Could you check a few things on this model? Use its own coordinates, in mm. Give positions to 0.01 mm unless a question says otherwise; leave off trailing zeros. Write each loop counter-clockwise with the first axis right and the second up, starting at its lowest first coordinate (ties: lowest second). Pieces come first, ordered by that corner, then holes. Notation, with made-up numbers: (-15.75, -15) - (31.25, -15) arc R26 cw to (31.25, 19) - close; hole circle Ø2 at (85, 22). An arc over 180 degrees is marked (long way). Answer in a Markdown table with one row per item.
from build123d import *

# Parameters (mm, degrees)
F0_W     = 175
F0_H     = 40
F1_DEPTH = 15
F3_DEPTH = 50.8
F5_DEPTH = 0.001


# Not quite as in the source:
# - a feature names something its author has since deleted; it is built from what else it names


with BuildPart() as f1:
    # F0 (on Top) → F1 (new body, symmetric)
    with BuildSketch(Plane.XY):
        Rectangle(F0_W, F0_H)
    extrude(amount=F1_DEPTH, both=True)

    # F2 (on face) → F3 (cut)
    with BuildSketch(Plane.XZ.offset(20)):
        with BuildLine():
            ThreePointArc((-87.5, 0), (-83.1066017178, 10.6066017178), (-72.5, 15))
            Line((-72.5, 15), (-87.5, 15))
            Line((-87.5, 15), (-87.5, 0))
        make_face()
        with BuildLine():
            Line((-87.5, -15), (-72.5, -15))
            ThreePointArc((-72.5, -15), (-83.1066017178, -10.6066017178), (-87.5, 0))
            Line((-87.5, 0), (-87.5, -15))
        make_face()
        with BuildLine():
            ThreePointArc((87.5, 0), (83.1066017178, -10.6066017178), (72.5, -15))
            Line((72.5, -15), (87.5, -15))
            Line((87.5, -15), (87.5, 0))
        make_face()
        with BuildLine():
            Line((87.5, 15), (72.5, 15))
            ThreePointArc((72.5, 15), (83.1066017178, 10.6066017178), (87.5, 0))
            Line((87.5, 0), (87.5, 15))
        make_face()
    extrude(amount=-F3_DEPTH, mode=Mode.SUBTRACT)

    # F4 (on face) → F5 (join)
    with BuildSketch(Plane.XZ.offset(20)):
        with BuildLine():
            Line((72, 12.5), (-72, 12.5))
            ThreePointArc((-72, 12.5), (-84.5, 0), (-72, -12.5))
            Line((-72, -12.5), (0, -12.5))
            Line((0, -12.5), (72, -12.5))
            ThreePointArc((72, -12.5), (84.5, 0), (72, 12.5))
        make_face()
    extrude(amount=F5_DEPTH)


solid = f1.part
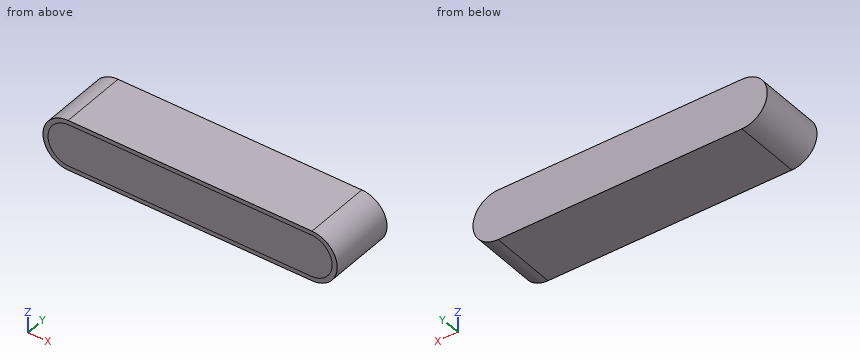
1) Will these pins go through, and if not, where does the flat tip stop? P1, Ø1, axis at y = 10, z = -4.5, coming from the -X side; P2, Ø5, axis at y = -2.5, z = 0.5, coming from the -X side; P3, Ø1.5, axis at y = 12.5, z = -3, coming from the -X side; P4, Ø4, axis at y = -7, z = -6, coming from the +X side.
Check values:
| item | result |
|---|---|
| P1 | stops at x = -86.96 |
| P2 | stops at x = -87.5 |
| P3 | stops at x = -87.33 |
| P4 | stops at x = 86.96 |
2) If I drill on line 1 (X direction, y = 13.5, z = 0.75); line 2 (Y direction, x = 15, z = 13.75); line 3 (X direction, y = -9, z = -3.75), over which ranges is the centre line in solid material (lowest first)?
Check values:
| item | result |
|---|---|
| line 1 | x = -87.48 to 87.48 |
| line 2 | y = -20 to 20 |
| line 3 | x = -87.02 to 87.02 |
3) Imagine slicing it at A-A (y = -15). List the corners of the cut face in (x, z) for me, then the cut area to 3 significant figures.
Check values:
| item | result |
|---|---|
| outline | (-72.5, -15) - (72.5, -15) arc R15 ccw to (72.5, 15) - (-72.5, 15) arc R15 ccw to start |
| area | 5,060 mm2 |
